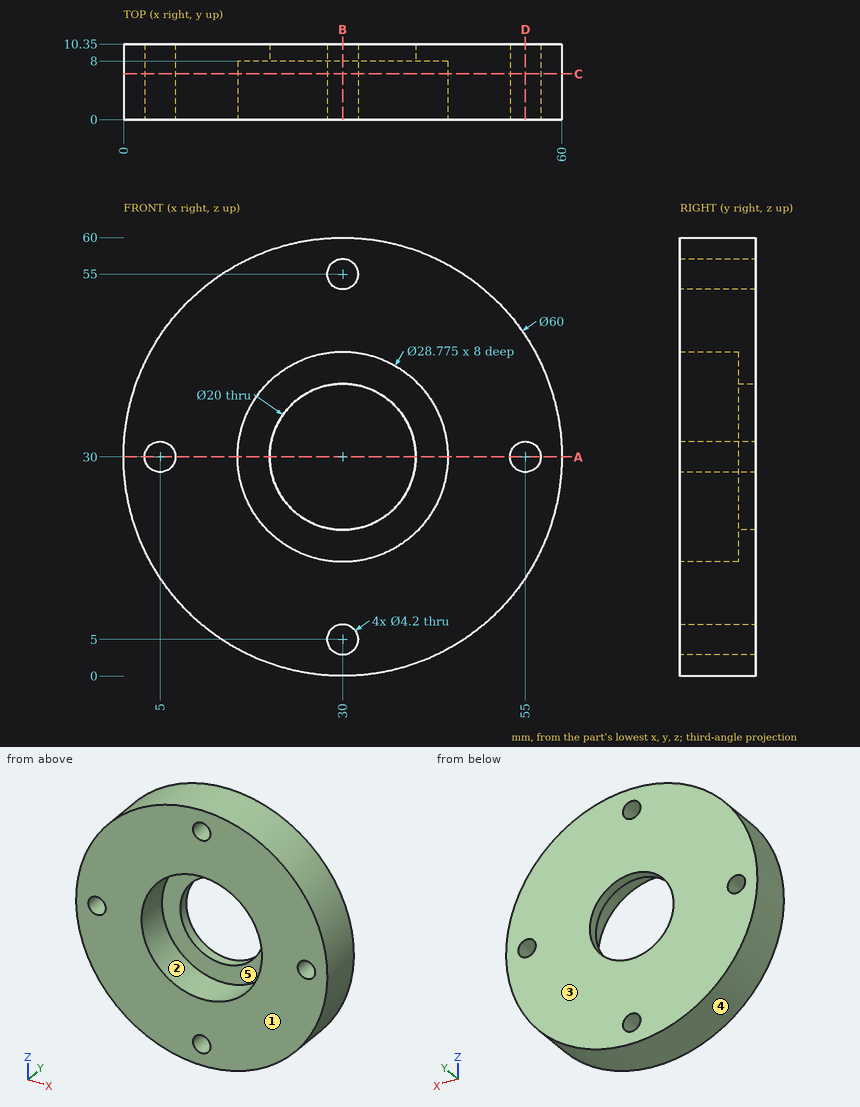
Study the drawing (mm; zero at the part's minimum x, y, z) and answer. A direction names the side the tool comes from. Give positions to 0.01 mm unless a question says otherwise; leave off trailing zeros. Order: outer loops, then holes, each group sorted by start corner. A loop starts at its lowest first (then second) coordinate and runs counter-clockwise, first axis right, second up. Notation, with made-up numbers: (0, 4.5) -> (53, 4.5) arc R27 ccw to (53, 42.5) -> close; hole circle Ø5 at (89, 77). An arc over 180 degrees is marked (long way). Write item = value, one per line.
1. A cutting plane is placed at C-C, the plane y = 6.25. Write down the section's boundary in (x, z) (1 decimal).
Numbers:
outline = circle Ø60 at (30, 30); hole circle Ø4.2 at (5, 30); hole circle Ø28.8 at (30, 30); hole circle Ø4.2 at (30, 5); hole circle Ø4.2 at (30, 55); hole circle Ø4.2 at (55, 30)
2. A cutting plane is placed at A-A, the plane z = 30. Write down the section's boundary in (x, y).
Numbers:
outline = (0, 0) -> (2.9, 0) -> (2.9, 10.35) -> (0, 10.35) -> close; (7.1, 0) -> (15.61, 0) -> (15.61, 8) -> (20, 8) -> (20, 10.35) -> (7.1, 10.35) -> close; (40, 8) -> (44.39, 8) -> (44.39, 0) -> (52.9, 0) -> (52.9, 10.35) -> (40, 10.35) -> close; (57.1, 0) -> (60, 0) -> (60, 10.35) -> (57.1, 10.35) -> close
3. A cutting plane is placed at D-D, the plane x = 55. Write down the section's boundary in (y, z), and give its area (3 significant figures).
Numbers:
outline = (0, 13.42) -> (10.35, 13.42) -> (10.35, 27.9) -> (0, 27.9) -> close; (0, 32.1) -> (10.35, 32.1) -> (10.35, 46.58) -> (0, 46.58) -> close
area = 300 mm²
4. Straight lines are drawn through the part: line 1 along X through (y, z) = (9.3, 30); line 2 along X through (y, z) = (3, 30); line 3 along X through (y, z) = (8.25, 5.5). For each, find the intervals that lie inside material, in ascending order.
Numbers:
line_1 = 0 to 2.9, 7.1 to 20, 40 to 52.9, 57.1 to 60
line_2 = 0 to 2.9, 7.1 to 15.61, 44.39 to 52.9, 57.1 to 60
line_3 = 12.69 to 27.96, 32.04 to 47.31
5. The mould has two halves that part along X. Classify the marked faces 3, 4 and 5: +X half, -X half, draft (parallel to the pull), parting line (faces both ways), or undercut.
Numbers:
face_3 = draft
face_4 = parting line
face_5 = undercut
6. Given pin 1 (1 mm diameter, centred on y = 5.5, z = 43, fed in from +X); pin 2 (3.5 mm diameter, centred on x = 30, z = 55, fed in from +Y); pin 3 (23 mm diameter, centred on x = 30, z = 30, fed in from -Y), each flat-ended and moving along its own axis, determine where each tip first touches the part or whether it passes through.
Numbers:
pin_1 = 57.27
pin_2 = through
pin_3 = 8
7. A cutting plane is placed at B-B, the plane x = 30. Write down the section's boundary in (y, z), and give its area (3 significant figures).
Numbers:
outline = (0, 0) -> (10.35, 0) -> (10.35, 2.9) -> (0, 2.9) -> close; (0, 7.1) -> (10.35, 7.1) -> (10.35, 20) -> (8, 20) -> (8, 15.61) -> (0, 15.61) -> close; (0, 44.39) -> (8, 44.39) -> (8, 40) -> (10.35, 40) -> (10.35, 52.9) -> (0, 52.9) -> close; (0, 57.1) -> (10.35, 57.1) -> (10.35, 60) -> (0, 60) -> close
area = 257 mm²
8. For the marked faces 1 and 2, determine the directions among +Z, -Z, +X, -X, +Y, -Y from which every point of the face is accessible in a straight line to the end or side of a thin tool.
Numbers:
face_1 = +Z, -Z, +X, -X, -Y
face_2 = -Y
